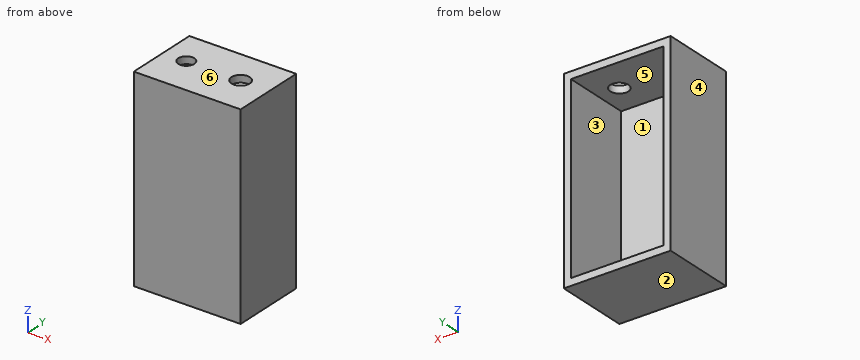
```python
from build123d import *

# Parameters (mm, degrees)
SKETCH_1_W          = 30
SKETCH_1_H          = 55
EXTRUDE_1_DEPTH     = 21
SKETCH_2_W          = 26
SKETCH_2_H          = 51
CUT_EXTRUDE_1_DEPTH = 19
SKETCH_3_R          = 2.2671126
SKETCH_3_R_2        = 2.57383576
CUT_EXTRUDE_2_DEPTH = 3


with BuildPart() as part:
    # Эскиз1 → Бобышка-Вытянуть1 (new body)
    with BuildSketch(Plane(origin=(0, 0, 0), x_dir=(1, 0, 0), z_dir=(0, 1, 0))):
        with Locations((15, 27.5)):
            Rectangle(SKETCH_1_W, SKETCH_1_H)
    extrude(amount=EXTRUDE_1_DEPTH)

    # Эскиз2 → Вырез-Вытянуть1 (cut)
    with BuildSketch(Plane(origin=(0, 21, 0), x_dir=(1, 0, 0), z_dir=(0, 1, 0))):
        with Locations((15, 27.5)):
            Rectangle(SKETCH_2_W, SKETCH_2_H)
    extrude(amount=-CUT_EXTRUDE_1_DEPTH, mode=Mode.SUBTRACT)

    # Эскиз3 → Вырез-Вытянуть2 (cut)
    with BuildSketch(Plane.XY):
        with Locations((6.524092584, 11.054705983)):
            Circle(SKETCH_3_R)
        with Locations((21.789601228, 11.054705983)):
            Circle(SKETCH_3_R_2)
    extrude(amount=-CUT_EXTRUDE_2_DEPTH, mode=Mode.SUBTRACT)


solid = part.part
```
Could you check a few things on this model? Use its own coordinates, in mm. Face numbers are marked on the shaded views. A direction names the side the tool comes from. Coordinates: 2 decimals unless noted, no trailing zeros. Write each loop counter-clockwise with the first axis right and the second up, starting at its lowest first coordinate (ties: lowest second). Pieces come first, ordered by that corner, then holes. Notation, with made-up numbers: (74.25, -16) -> (95.25, -16) arc R25 cw to (95.25, 10) -> close; hole circle Ø4 at (-33, 34.5). An arc over 180 degrees is marked (long way). Write item = value, one per line. Start each with the question number.
(1) I need wall thicknesses on line 1 (X direction, y = 15, z = -26.5); line 2 (Z direction, x = 5.5, y = 19.25); line 3 (Y direction, x = 11, z = -7). Which ranges of each line are inside material? Lowest first, please. Write a range as [from, to].
(2) I want a section at B-B (x = 22.25). Please give me the cut outline in (y, z).
(3) I want a section at D-D (x = 27). Please give me the cut outline in (y, z), plus the area to 3 significant figures.
(4) We'd pull the mould along Z, two halves only. Please class the marked faces 3, 4, 5 and 6: released by +Z, released by -Z, zero draft, split by the parting line, or undercut.
(5) I want a section at C-C (z = -43). Please give me the cut outline in (x, y).
(6) I want a section at A-A (y = 4). Please give me the cut outline in (x, z).
(7) Which directions (+Z, -Z, +X, -X, +Y, -Y) give clear straight access to the entire face, cutting with the end or side of a thin tool? Please do the marked faces 1 and 2.
(8) Will these pins go through, and if not, where does the flat tip stop? pin 1 (8 mm diameter, centred on x = 13.5, z = -16, fed in from +Y); pin 2 (9.5 mm diameter, centred on y = 8.5, z = -21, fed in from -X).
Result set:
q1.line_1 = [0, 2], [28, 30]
q1.line_2 = [-55, -53], [-2, 0]
q1.line_3 = [0, 2]
q2.outline = (0, -55) -> (21, -55) -> (21, -53) -> (2, -53) -> (2, -2) -> (8.52, -2) -> (8.52, 0) -> (0, 0) -> close; (13.59, -2) -> (21, -2) -> (21, 0) -> (13.59, 0) -> close
q3.outline = (0, -55) -> (21, -55) -> (21, -53) -> (2, -53) -> (2, -2) -> (21, -2) -> (21, 0) -> (0, 0) -> close
q3.area = 186 mm2
q4.face_3 = undercut
q4.face_4 = zero draft
q4.face_5 = undercut
q4.face_6 = released by +Z
q5.outline = (0, 0) -> (30, 0) -> (30, 21) -> (28, 21) -> (28, 2) -> (2, 2) -> (2, 21) -> (0, 21) -> close
q6.outline = (0, -55) -> (30, -55) -> (30, 0) -> (0, 0) -> close; hole (2, -53) -> (28, -53) -> (28, -2) -> (2, -2) -> close
q7.face_1 = +Y
q7.face_2 = -Z, +X, -X, +Y, -Y
q8.pin_1 = 2
q8.pin_2 = 0
